from build123d import *

# Parameters (mm, degrees)
SKETCH1_W                                            = 60
SKETCH1_H                                            = 60
BOSS_EXTRUDE1_DEPTH                                  = 10
M4_TAPPED_HOLE1_D                                    = 3.3
M4_TAPPED_HOLE1_DEPTH                                = 7.108579979
M4_TAPPED_HOLE1_TIP                                  = 0.991420021
CSK_FOR_M4_HEX_SOCKET_COUNTERSUNK_CAP_SC_D           = 4.5
CSK_FOR_M4_HEX_SOCKET_COUNTERSUNK_CAP_SC_CSINK_D     = 8.96
CSK_FOR_M4_HEX_SOCKET_COUNTERSUNK_CAP_SC_CSINK_ANGLE = 90
M4_TAPPED_HOLE2_D                                    = 3.3
M4_TAPPED_HOLE2_DEPTH                                = 8
M4_TAPPED_HOLE2_TIP                                  = 0.991420021
FILLET1_R                                            = 5


with BuildPart() as part:
    # Sketch1 → Boss-Extrude1 (new body)
    with BuildSketch(Plane.XY):
        with Locations((30, 30)):
            Rectangle(SKETCH1_W, SKETCH1_H)
    extrude(amount=BOSS_EXTRUDE1_DEPTH)

    # M4 Tapped Hole1
    with Locations(Plane.XY.offset(10)):
        with Locations((5, 55), (55, 55), (55, 5), (5, 5)):
            Hole(M4_TAPPED_HOLE1_D / 2, depth=M4_TAPPED_HOLE1_DEPTH)
            with Locations((0, 0, -(M4_TAPPED_HOLE1_DEPTH + M4_TAPPED_HOLE1_TIP / 2))):  # 118° drill point
                Cone(0, M4_TAPPED_HOLE1_D / 2, M4_TAPPED_HOLE1_TIP, mode=Mode.SUBTRACT)

    # CSK for M4 Hex Socket Countersunk Cap Screw1 (through all)
    with Locations(Plane.XY.offset(10)):
        with Locations((30, 40), (30, 15)):
            CounterSinkHole(CSK_FOR_M4_HEX_SOCKET_COUNTERSUNK_CAP_SC_D / 2, CSK_FOR_M4_HEX_SOCKET_COUNTERSUNK_CAP_SC_CSINK_D / 2, counter_sink_angle=CSK_FOR_M4_HEX_SOCKET_COUNTERSUNK_CAP_SC_CSINK_ANGLE)

    # M4 Tapped Hole2
    with Locations(Plane(origin=(0, 0, 0), x_dir=(-1, 0, 0), z_dir=(0, -1, 0))):
        with Locations((-30, -5), (-14, -5), (-46, -5)):
            Hole(M4_TAPPED_HOLE2_D / 2, depth=M4_TAPPED_HOLE2_DEPTH)
            with Locations((0, 0, -(M4_TAPPED_HOLE2_DEPTH + M4_TAPPED_HOLE2_TIP / 2))):  # 118° drill point
                Cone(0, M4_TAPPED_HOLE2_D / 2, M4_TAPPED_HOLE2_TIP, mode=Mode.SUBTRACT)

    # Fillet1
    fillet1_edges = [part.edges().sort_by_distance(p)[0] for p in [
        (0, 60, 5),
        (60, 60, 5),
        (60, 0, 5),
        (0, 0, 5),
    ]]
    fillet(fillet1_edges, radius=FILLET1_R)


solid = part.part
Design review of the part built by this model. Coordinates are the model's own, in mm. A direction names the side the tool comes from. Round coordinates to 2 decimals unless told otherwise and drop trailing zeros. Loops run counter-clockwise (first coordinate to the right, second up) from the corner with the lowest first, then second, coordinate; pieces in that order, holes last. Notation, with made-up numbers: (46, 0.25) - (86, 0.25) arc R13 ccw to (86, 9.25) - close; hole circle Ø11 at (67.25, 76.5). An arc over 180 degrees is marked (long way). One line per item, written item: value. Start each with the question number.
1) Consider section A-A on y = 15. Give the boundary of the cut face in (x, z).
2) To check wall thickness, follow L1, parallel to Y at x = 5, z = 5.5; L2, parallel to Y at x = 30, z = 2.5; L3, parallel to Z at x = 14, y = 3. State the ranges of each line that lie inside material, in increasing order. Write a range as from..to.
3) For faces 1 (the cylindrical face through (6.31, 4, 6.4)), 2 (the cylindrical face through (28.69, 4.06, 6)), 3 (the cylindrical face through (58, 59, 5)), list the 3-axis set-ups (+Z, -Z, +X, -X, +Y, -Y) from which the entire face can be reached by the end or side of a thin tool; tool diameter is ignored.
4) Consider section B-B on z = 5.75. Give the number of separate pieces and of enclosed holes in the cut face, then the cut area to 3 significant figures.
5) Draft analysis for pull direction Y (two halves, no side actions). For faces 4 (the conical face through (14.23, 8.82, 5.17)), 5 (the flat face through (0, 30, 5)), 6 (the cylindrical face through (56.65, 55.07, 6.4)), state which applies: +Y half, -Y half, draft (parallel to the pull), parting line (faces both ways), or undercut.
6) Insertion check: pin 1 Ø3.5 at (x, y) = (30, 15) entering from -Z; pin 2 Ø2.5 at (x, z) = (30, 5) entering from -Y. Each pin has a flat end and moves straight along its axis. Give the tip position at first contact, or say it passes through.
Reported:
1. outline: (0, 0) - (27.75, 0) - (27.75, 7.77) - (25.52, 10) - (0, 10) - close; (32.25, 0) - (60, 0) - (60, 10) - (34.48, 10) - (32.25, 7.77) - close
2. L1: y = 0..3.35, 6.65..53.35, 56.65..60
2. L2: y = 0..12.75, 17.25..37.75, 42.25..60
2. L3: z = 0..3.35, 6.65..10
3. face 1: +Z
3. face 2: -Y
3. face 3: +Z, -Z, +X, +Y
4. separate pieces: 1
4. enclosed holes: 6
4. area: 3,440 mm^2
5. face 4: -Y half
5. face 5: draft
5. face 6: undercut
6. pin 1: passes through
6. pin 2: stops at y = 8.24
